Read the model definition and answer for the solid it produces. Units are mm, in the model's axes. A direction names the side the tool comes from. Round coordinates to 2 decimals unless told otherwise and drop trailing zeros. Loops run counter-clockwise (first coordinate to the right, second up) from the corner with the lowest first, then second, coordinate; pieces in that order, holes last. Notation, with made-up numbers: M -21.75,56 L 1.25,56 A21 cw 1.25,82 Z; hole C -28.75,40 d5. An arc over 180 degrees is marked long. Write each question's results on one line, items separated by ' | '.
```python
from build123d import *

# Parameters (mm, degrees)
BOSS_EXTRUDE1_DEPTH = 26
RIB1_REACH          = 65.738
SKETCH3_WALL_W      = 172.022520638
SKETCH3_WALL_H      = 8


with BuildPart() as part:
    # Sketch2 → Boss-Extrude1 (new, symmetric)
    with BuildSketch(Plane.XY):
        with BuildLine():
            Line((-23, 44.5), (-15, 44.5))
            ThreePointArc((-15, 44.5), (0, 29.5), (15, 44.5))
            Line((15, 44.5), (23, 44.5))
            ThreePointArc((23, 44.5), (17.783419244, 29.914047854), (4.5, 21.944512863))
            Line((4.5, 21.944512863), (4.5, 4.5))
            Line((4.5, 4.5), (37.5, 4.5))
            Line((37.5, 4.5), (37.5, -4.5))
            Line((37.5, -4.5), (-37.5, -4.5))
            Line((-37.5, -4.5), (-37.5, 4.5))
            Line((-37.5, 4.5), (-4.5, 4.5))
            Line((-4.5, 4.5), (-4.5, 21.944512863))
            ThreePointArc((-4.5, 21.944512863), (-17.783419244, 29.914047854), (-23, 44.5))
        make_face()
    extrude(amount=BOSS_EXTRUDE1_DEPTH, both=True)

    # Sketch3 wall → Rib1 (add, up to next)
    with BuildSketch(Plane(origin=(30.25, 24.5, 0), x_dir=(0.340799323621, -0.940136065162, 0), z_dir=(0.940136065162, 0.340799323621, 0)), mode=Mode.PRIVATE) as rib1_sk1:
        Rectangle(SKETCH3_WALL_W, SKETCH3_WALL_H)
    rib1_tool1 = extrude(rib1_sk1.sketch, amount=-RIB1_REACH, mode=Mode.PRIVATE) - part.part
    rib1 = rib1_tool1.solids().sort_by_distance((30.25, 24.5, 0))[0]
    add(rib1)

    # Mirror1: Rib1 across plane
    add(rib1.mirror(Plane(origin=(0, 0, 0), x_dir=(0, 0, 1), z_dir=(1, 0, 0))))


solid = part.part
```
1. Find section D-D, the plane y = 18. Give the vertices of the cut face in (x, z), then the cut area to 3 significant figures.
Completed:
outline: M -32.61,-4 L -4.5,-4 L -4.5,-26 L 4.5,-26 L 4.5,-4 L 32.61,-4 L 32.61,4 L 4.5,4 L 4.5,26 L -4.5,26 L -4.5,4 L -32.61,4 Z | area: 918 mm2
2. Find section B-B, the plane z = -10. Give the vertices of the cut face in (x, y), then the cut area to 3 significant figures.
Completed:
outline: M -37.5,-4.5 L 37.5,-4.5 L 37.5,4.5 L 4.5,4.5 L 4.5,21.94 A23 ccw 23,44.5 L 15,44.5 A15 cw -15,44.5 L -23,44.5 A23 ccw -4.5,21.94 L -4.5,4.5 L -37.5,4.5 Z | area: 1,310 mm2
3. Find the intervals of material crossed by L1, parallel to Y at x = 13.5, z = -4.5; L2, parallel to Y at x = -16, z = -8.5; L3, parallel to X at y = 33, z = -2, in increasing order.
Completed:
L1: y = -4.5 to 4.5, 25.88 to 37.96 | L2: y = -4.5 to 4.5, 27.98 to 44.5 | L3: x = -27.17 to -9.63, 9.63 to 27.17
4. Find section C-C, the plane x = -29. Give the vertices of the cut face in (y, z).
Completed:
outline: M -4.5,-26 L 4.5,-26 L 4.5,-4 L 27.95,-4 L 27.95,4 L 4.5,4 L 4.5,26 L -4.5,26 Z
5. Find section A-A, the plane y = 31. Give the vertices of the cut face in (x, z).
Completed:
outline: M -27.89,-4 L -18.62,-4 L -18.62,-26 L -6.54,-26 L -6.54,26 L -18.62,26 L -18.62,4 L -27.89,4 Z; M 6.54,-26 L 18.62,-26 L 18.62,-4 L 27.89,-4 L 27.89,4 L 18.62,4 L 18.62,26 L 6.54,26 Z
6. Determine the mould class of faces 4 (the face through (-37.5, 0, 0)), 5 (the face through (-0.33, 29.504, 0.364)), 6 (the face through (21, 4.5, -15)) for opening direction X: released by +X, released by -X, zero draft, split by the parting line, or undercut.
Completed:
face 4: released by -X | face 5: undercut | face 6: zero draft
7. Which of the six approach directions +Z, -Z, +X, -X, +Y, -Y give full straight-line access (tool end or side, diameter ignored) to faces 1 (the face through (-21, 16, 4)), 2 (the face through (17.923, 30.086, 15.154)), 3 (the face through (-4.5, 13, -15))?
Completed:
face 1: +Z, -X | face 2: +Z, +X | face 3: -Z, -X
8. Given P1, Ø8.5, axis at y = 10, z = -12.5, coming from the -X side; P2, Ø10, axis at x = -22.5, y = 25.5, coming from the -Z side; P3, Ø16.5, axis at x = -26.5, y = 26.5, coming from the +Z side, each flat-ended and moving along its own axis, determine where each tip first touches the part or whether it passes through.
Completed:
P1: stops at x = -4.5 | P2: stops at z = -4 | P3: stops at z = 4
